from build123d import *

# Parameters (mm, degrees)
SKETCH1_W                 = 83
SKETCH1_H                 = 83
BOSS_EXTRUDE1_DEPTH       = 6
SKETCH2_R                 = 1.5
CUT_EXTRUDE1_DEPTH        = 118.532974097
SKETCH4_R                 = 1.5
CUT_EXTRUDE4_DEPTH        = 3
BOSS_EXTRUDE2_START       = -3
BOSS_EXTRUDE2_OUTLINE_R   = 1.5
BOSS_EXTRUDE2_DEPTH       = 3
BOSS_EXTRUDE2_2_OUTLINE_W = 50
BOSS_EXTRUDE2_2_OUTLINE_H = 32
BOSS_EXTRUDE2_2_DEPTH     = 22
SKETCH6_W                 = 44
SKETCH6_H                 = 26
CUT_EXTRUDE5_DEPTH        = 25
CUT_EXTRUDE14_DEPTH       = 22
CUT_EXTRUDE15_DEPTH       = 121.012499349
FILLET2_R                 = 5


# Read off the part's stored shape, not the designer's step: Boss-Extrude2
with BuildPart() as part:
    # Sketch1 → Boss-Extrude1 (new body)
    with BuildSketch(Plane(origin=(0, 0, 0), x_dir=(1, 0, 0), z_dir=(0, 1, 0))):
        with Locations((41.5, 41.5)):
            Rectangle(SKETCH1_W, SKETCH1_H)
    extrude(amount=BOSS_EXTRUDE1_DEPTH)

    # Sketch2 → Cut-Extrude1 (cut, through all)
    with BuildSketch(Plane(origin=(0, 6, 0), x_dir=(1, 0, 0), z_dir=(0, 1, 0))):
        with Locations(Location((6, 71, 0), (0, 0, 270))):
            Circle(SKETCH2_R)
        with Locations(Location((6, 12, 0), (0, 0, 270))):
            Circle(SKETCH2_R)
        with Locations(Location((77, 12, 0), (0, 0, 270))):
            Circle(SKETCH2_R)
        with Locations(Location((77, 71, 0), (0, 0, 270))):
            Circle(SKETCH2_R)
    extrude(amount=-CUT_EXTRUDE1_DEPTH, mode=Mode.SUBTRACT)

    # Sketch4 → Cut-Extrude4 (cut)
    with BuildSketch(Plane(origin=(0, 6, 0), x_dir=(1, 0, 0), z_dir=(0, 1, 0))):
        Polygon((13, 15), (13, 9), (3, 9), (3, 21), (8, 21), align=None)
        with Locations(Location((6, 12, 0), (0, 0, 270))):
            Circle(SKETCH4_R, mode=Mode.SUBTRACT)
    cut_extrude4 = extrude(amount=-CUT_EXTRUDE4_DEPTH, mode=Mode.SUBTRACT)

    # Mirror2: Cut-Extrude4 across plane
    add(cut_extrude4.mirror(Plane.XY.offset(-41.5)), mode=Mode.SUBTRACT)

    # Boss-Extrude2 outline → Boss-Extrude2 (cut)
    # profile 1 of 2: a face of its own
    with BuildSketch(Plane(origin=(0, 6, 0), x_dir=(1, 0, 0), z_dir=(0, 1, 0)).offset(BOSS_EXTRUDE2_START)):
        Polygon((75, 21), (70, 15), (70, 9), (80, 9), (80, 21), align=None)
        with Locations((77, 12)):
            Circle(BOSS_EXTRUDE2_OUTLINE_R, mode=Mode.SUBTRACT)
    # profile 2 of 2: a face of its own
    with BuildSketch(Plane(origin=(0, 6, 0), x_dir=(1, 0, 0), z_dir=(0, 1, 0)).offset(BOSS_EXTRUDE2_START)):
        Polygon((75, 62), (80, 62), (80, 74), (70, 74), (70, 68), align=None)
        with Locations((77, 71)):
            Circle(BOSS_EXTRUDE2_OUTLINE_R, mode=Mode.SUBTRACT)
    extrude(amount=BOSS_EXTRUDE2_DEPTH, mode=Mode.SUBTRACT)

    # Boss-Extrude2 2 outline → Boss-Extrude2 2 (add)
    with BuildSketch(Plane(origin=(0, 6, 0), x_dir=(1, 0, 0), z_dir=(0, 1, 0))):
        with Locations((49.5, 16)):
            Rectangle(BOSS_EXTRUDE2_2_OUTLINE_W, BOSS_EXTRUDE2_2_OUTLINE_H)
    extrude(amount=BOSS_EXTRUDE2_2_DEPTH)

    # Sketch6 → Cut-Extrude5 (cut)
    with BuildSketch(Plane(origin=(0, 28, 0), x_dir=(1, 0, 0), z_dir=(0, 1, 0))):
        with Locations((49.5, 16)):
            Rectangle(SKETCH6_W, SKETCH6_H)
    extrude(amount=-CUT_EXTRUDE5_DEPTH, mode=Mode.SUBTRACT)

    # Sketch8 → Cut-Extrude14 (cut)
    with BuildSketch(Plane(origin=(0, 28, 0), x_dir=(1, 0, 0), z_dir=(0, 1, 0))):
        with BuildLine():
            Line((74.5, 9), (74.5, 17.454356057))
            ThreePointArc((74.5, 17.454356057), (72.718007844, 16.202920792), (71.5, 14.397915762))
            Line((71.5, 14.397915762), (71.5, 9.602084238))
            ThreePointArc((71.5, 9.602084238), (71.64345769, 9.296769621), (71.803847577, 9))
            Line((71.803847577, 9), (74.5, 9))
        make_face()
        with BuildLine():
            Line((74.5, 6.545643943), (74.5, 9))
            Line((74.5, 9), (71.803847577, 9))
            ThreePointArc((71.803847577, 9), (72.960983233, 7.563070481), (74.5, 6.545643943))
        make_face()
    extrude(amount=-CUT_EXTRUDE14_DEPTH, mode=Mode.SUBTRACT)

    # Sketch13 → Cut-Extrude15 (cut, through all)
    with BuildSketch(Plane(origin=(0, 3, 0), x_dir=(1, 0, 0), z_dir=(0, 1, 0))):
        Polygon((71.5, 9), (80, 9), (80, 21), (75, 21), (71.5, 16.8), (71.5, 29), (27.5, 29), (27.5, 3), (71.5, 3), align=None)
    extrude(amount=CUT_EXTRUDE15_DEPTH, mode=Mode.SUBTRACT)

    # Fillet2
    fillet2_edges = [part.edges().sort_by_distance(p)[0] for p in [
        (74.5, 17, -32),
        (24.5, 17, -32),
    ]]
    fillet(fillet2_edges, radius=FILLET2_R)


solid = part.part
Verification items for the finished model (mm, model axes). A direction names the side the tool comes from. Give positions to 0.01 mm unless a question says otherwise; leave off trailing zeros. Loops run counter-clockwise (first coordinate to the right, second up) from the corner with the lowest first, then second, coordinate; pieces in that order, holes last.
1) Thickness scan on line 1 along X through (y, z) = (1.6, -71); line 2 along Z through (x, y) = (77, 2.25); line 3 along Z through (x, y) = (33, 14.25). Record the ranges inside material, lowest first.
2) Sectioned sample at C-C, the plane x = 52. Enter the section's corners in (y, z).
3) Sectioned sample at D-D, the plane y = 25.5. Enter the section's corners in (x, z).
4) Sectioned sample at A-A, the plane z = -12. Enter the section's corners in (x, y), then the cut area to 4 significant figures.
5) Set-up check for faces 1 (the cylindrical face through (73.07, 17.15, -30.5)), 2 (the flat face through (10.5, 4.5, -65)), 3 (the cylindrical face through (6.07, 1.52, -13.5)): record each of +Z, -Z, +X, -X, +Y, -Y from which the full face is reachable in a straight line by a thin tool's end or side.
6) Sectioned sample at B-B, the plane x = 77. Enter the section's corners in (y, z).
7) Depth check by flat-ended pin: pin 1 Ø10 at (x, y) = (19, 20) entering from +Z; pin 2 Ø0.9 at (y, z) = (4, -68) entering from -X; pin 3 Ø5 at (x, y) = (42, 21.5) entering from -Z; pin 4 Ø1 at (x, z) = (58.5, -25.5) entering from +Y. Enter the tip coordinate at first touch or a pass-through.
8) Draft check along Z on faces 4 (the flat face through (75, 4, -74)), 5 (the flat face through (74.5, 17, -24)), 6 (the flat face through (50, 11, 0)), 7 (the flat face through (53, 3, -16)). Enter one of: pulls with the +Z half, pulls with the -Z half, needs draft (parallel to the pull), parting line crosses it, or undercut.
Answers:
1. line 1: x = 0 to 4.5, 7.5 to 75.5, 78.5 to 83
1. line 2: z = -83 to -72.5, -69.5 to -13.5, -10.5 to 0
1. line 3: z = -32 to -29, -3 to 0
2. outline: (0, -83) - (6, -83) - (6, -32) - (28, -32) - (28, -29) - (3, -29) - (3, -3) - (28, -3) - (28, 0) - (0, 0) - close
3. outline: (24.5, -27) arc R5 ccw to (29.5, -32) - (69.5, -32) arc R5 ccw to (74.5, -27) - (74.5, -20.4) - (71.5, -16.8) - (71.5, -29) - (27.5, -29) - (27.5, -3) - (71.5, -3) - (71.5, -9) - (71.8, -9) arc R6 cw to (74.5, -6.55) - (74.5, 0) - (24.5, 0) - close
4. outline: (0, 0) - (4.5, 0) - (4.5, 3) - (3, 3) - (3, 6) - (0, 6) - close; (7.5, 0) - (75.5, 0) - (75.5, 3) - (27.5, 3) - (27.5, 28) - (24.5, 28) - (24.5, 6) - (13, 6) - (13, 3) - (7.5, 3) - close; (78.5, 0) - (83, 0) - (83, 6) - (80, 6) - (80, 3) - (78.5, 3) - close
4. area: 358.5 mm2
5. face 1: -Z, +X, +Y
5. face 2: +Y
5. face 3: +Y, -Y
6. outline: (0, -83) - (6, -83) - (6, -74) - (3, -74) - (3, -72.5) - (0, -72.5) - close; (0, -69.5) - (3, -69.5) - (3, -62) - (6, -62) - (6, -21) - (3, -21) - (3, -13.5) - (0, -13.5) - close; (0, -10.5) - (3, -10.5) - (3, -9) - (6, -9) - (6, 0) - (0, 0) - close
7. pin 1: passes through
7. pin 2: stops at x = 0
7. pin 3: stops at z = -32
7. pin 4: stops at y = 3
8. face 4: undercut
8. face 5: needs draft
8. face 6: pulls with the +Z half
8. face 7: undercut
